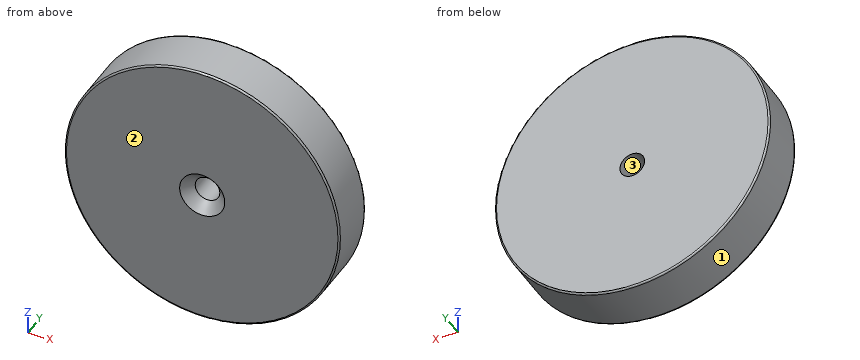
```python
from build123d import *

# Parameters (mm, degrees)
F0_R           = 16.75
F1_DEPTH       = 6
F3_D           = 3
F3_CSINK_D     = 5.5
F3_CSINK_ANGLE = 90
F4_R           = 0.2


with BuildPart() as f1:
    # F0 (on Front) → F1 (new body)
    with BuildSketch(Plane.XZ):
        Circle(F0_R)
    extrude(amount=F1_DEPTH)

    # F3 (through all)
    with Locations(Plane.XZ.offset(6)):
        with Locations((0, 0)):
            CounterSinkHole(F3_D / 2, F3_CSINK_D / 2, counter_sink_angle=F3_CSINK_ANGLE)

    # F4
    f4_edges = [f1.edges().sort_by_distance(p)[0] for p in [
        (-16.75, -6, 0),
        (-16.75, 0, 0),
    ]]
    fillet(f4_edges, radius=F4_R)


solid = f1.part
```
Read the model definition and answer for the solid it produces. Units are mm, in the model's axes. Face numbers are marked on the shaded views. Round coordinates to 2 decimals unless told otherwise and drop trailing zeros. Loops run counter-clockwise (first coordinate to the right, second up) from the corner with the lowest first, then second, coordinate; pieces in that order, holes last. Notation, with made-up numbers: (26, 65.5) -> (70, 65.5) arc R23 ccw to (70, 102.5) -> close; hole circle Ø11 at (45.25, 85). An arc over 180 degrees is marked (long way). One line per item, written item: value.
1) A cutting plane is placed at A-A (x = 0). Determine the outline of the cut face in (y, z).
Answer list:
outline: (-6, -16.55) arc R0.2 ccw to (-5.8, -16.75) -> (-0.2, -16.75) arc R0.2 ccw to (0, -16.55) -> (0, -1.5) -> (-4.75, -1.5) -> (-6, -2.75) -> close; (-6, 2.75) -> (-4.75, 1.5) -> (0, 1.5) -> (0, 16.55) arc R0.2 ccw to (-0.2, 16.75) -> (-5.8, 16.75) arc R0.2 ccw to (-6, 16.55) -> close
2) Consider L1, parallel to Z at x = 0, y = -1.15; L2, parallel to Z at x = -0.5, y = -0.75; L3, parallel to X at y = -3.95, z = -12.5. Determine where each line is inside the solid, lowest interval first. Write a range as [from, to].
Answer list:
L1: z = [-16.75, -1.5], [1.5, 16.75]
L2: z = [-16.74, -1.41], [1.41, 16.74]
L3: x = [-11.15, 11.15]
3) A cutting plane is placed at C-C (y = -2.55). Determine the outline of the cut face in (x, z).
Answer list:
outline: circle Ø33.5 at (0, 0); hole circle Ø3 at (0, 0)
4) A cutting plane is placed at B-B (z = 0). Determine the outline of the cut face in (x, y), and give its area (3 significant figures).
Answer list:
outline: (-16.75, -5.8) arc R0.2 ccw to (-16.55, -6) -> (-2.75, -6) -> (-1.5, -4.75) -> (-1.5, 0) -> (-16.55, 0) arc R0.2 ccw to (-16.75, -0.2) -> close; (1.5, -4.75) -> (2.75, -6) -> (16.55, -6) arc R0.2 ccw to (16.75, -5.8) -> (16.75, -0.2) arc R0.2 ccw to (16.55, 0) -> (1.5, 0) -> close
area: 181 mm²
5) The mould has two halves that part along X. Classify the marked faces 1, 2 and 3: pulls with the +X half, pulls with the -X half, needs draft (parallel to the pull), parting line crosses it, or undercut.
Answer list:
face 1: parting line crosses it
face 2: needs draft
face 3: undercut
6) Flat-ended cylindrical pins translate along their axes: P1, Ø1.5, axis at y = -1.5, z = -7, coming from the +X side; P2, Ø1.8, axis at x = 0, z = 0, coming from the +Y side; P3, Ø1, axis at y = -4, z = 7, coming from the +X side. Find the tip coordinate at first contact, or state that the pin passes through.
Answer list:
P1: stops at x = 15.54
P2: passes through
P3: stops at x = 15.44
